Geometry check sheet. Reference: the model listing, model coordinates, mm. Give positions to 0.01 mm unless a question says otherwise; leave off trailing zeros. Loops run counter-clockwise (first coordinate to the right, second up) from the corner with the lowest first, then second, coordinate; pieces in that order, holes last. Notation, with made-up numbers: (-35.75, 12.25) -> (-6.75, 12.25) arc R28 ccw to (-6.75, 33.25) -> close; hole circle Ø9 at (11, -8). An arc over 180 degrees is marked (long way). Write each question's results on one line, items separated by ' | '. Start each with the question number.
1) Scan lines: line 1 (X direction, y = 0, z = 2.3); line 2 (X direction, y = 4, z = 1.35); line 3 (X direction, y = -4.5, z = 0.6). Record each from-to range of solid material in increasing order. Write a range as from..to.
2) Depth check by flat-ended pin: pin 1 (0.9 mm diameter, centred on y = 2.5, z = 2, fed in from -X); pin 2 (1 mm diameter, centred on y = -4.5, z = 2, fed in from -X); pin 3 (0.9 mm diameter, centred on x = 4, z = 2, fed in from +Y). Enter the tip coordinate at first touch or a pass-through.
3) Sectioned sample at A-A on y = 0. Record the cut outline in (x, z).
4) Sectioned sample at B-B on z = 1. Record the cut outline in (x, y), then the cut area to 3 significant figures.
5) Sectioned sample at D-D on y = -4. Record the cut outline in (x, z), then the cut area to 3 significant figures.
6) Sectioned sample at C-C on y = 5.25. Record the cut outline in (x, z), then the cut area to 3 significant figures.
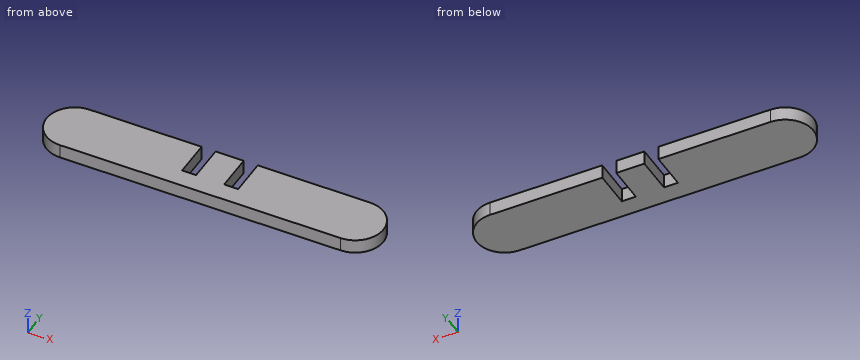
```python
from build123d import *

# Parameters (mm, degrees)
EXTRUDE_1_DEPTH     = 3
SKETCH_2_W          = 3
SKETCH_2_H          = 8
CUT_EXTRUDE_1_DEPTH = 4


with BuildPart() as part:
    # 草图1 → 凸台-拉伸1 (new body)
    with BuildSketch(Plane.XY):
        with BuildLine():
            Line((30, -6), (-30, -6))
            ThreePointArc((-30, -6), (-36, 0), (-30, 6))
            Line((-30, 6), (30, 6))
            ThreePointArc((30, 6), (36, 0), (30, -6))
        make_face()
    extrude(amount=EXTRUDE_1_DEPTH)

    # 草图2 → 切除-拉伸1 (cut)
    with BuildSketch(Plane.XY.offset(3)):
        with Locations((-4.5, 2)):
            Rectangle(SKETCH_2_W, SKETCH_2_H)
        with Locations((4.5, 2)):
            Rectangle(SKETCH_2_W, SKETCH_2_H)
    extrude(amount=-CUT_EXTRUDE_1_DEPTH, mode=Mode.SUBTRACT)


solid = part.part
```
Result:
1) line 1: -36..-6, -3..3, 6..36 | line 2: -34.47..-6, -3..3, 6..34.47 | line 3: -33.97..33.97
2) pin 1: x = -35.64 | pin 2: x = -34.47 | pin 3: y = -2
3) outline: (-36, 0) -> (-6, 0) -> (-6, 3) -> (-36, 3) -> close; (-3, 0) -> (3, 0) -> (3, 3) -> (-3, 3) -> close; (6, 0) -> (36, 0) -> (36, 3) -> (6, 3) -> close
4) outline: (-30, -6) -> (30, -6) arc R6 ccw to (30, 6) -> (6, 6) -> (6, -2) -> (3, -2) -> (3, 6) -> (-3, 6) -> (-3, -2) -> (-6, -2) -> (-6, 6) -> (-30, 6) arc R6 ccw to start | area: 785 mm^2
5) outline: (-34.47, 0) -> (34.47, 0) -> (34.47, 3) -> (-34.47, 3) -> close | area: 207 mm^2
6) outline: (-32.9, 0) -> (-6, 0) -> (-6, 3) -> (-32.9, 3) -> close; (-3, 0) -> (3, 0) -> (3, 3) -> (-3, 3) -> close; (6, 0) -> (32.9, 0) -> (32.9, 3) -> (6, 3) -> close | area: 179 mm^2
